Input: part model. Units: mm. Frame: model coordinates. A direction names the side the tool comes from. Give positions to 0.01 mm unless a question says otherwise; leave off trailing zeros. Write each loop counter-clockwise with the first axis right and the second up, starting at its lowest first coordinate (ties: lowest second). Pieces come first, ordered by that corner, then holes.
```python
from build123d import *

# Parameters (mm, degrees)
CROQUIS1_W                                     = 210
CROQUIS1_H                                     = 108
SALIENTE_EXTRUIR1_DEPTH                        = 103
CORTAR_EXTRUIR2_DEPTH                          = 108
REFRENTADO_PARA_TORNILLO_CON_CABEZA_2_COUNT    = 2
REFRENTADO_PARA_TORNILLO_CON_CABEZA_2_PITCH    = 76.278637259
REFRENTADO_PARA_TORNILLO_CON_CABEZA_3_COUNT    = 2
REFRENTADO_PARA_TORNILLO_CON_CABEZA_3_PITCH    = 109.392089664
REFRENTADO_PARA_TORNILLO_CON_CABEZA_4_COUNT    = 2
REFRENTADO_PARA_TORNILLO_CON_CABEZA_4_PITCH    = 78.410450701
REFRENTADO_PARA_TORNILLO_CON_CABEZA_5_AT_COUNT = 2
REFRENTADO_PARA_TORNILLO_CON_CABEZA_5_AT_PITCH = 74.028637259
REFRENTADO_PARA_TORNILLO_CON_CABEZA_6_COUNT    = 2
REFRENTADO_PARA_TORNILLO_CON_CABEZA_6_PITCH    = 111.845629414
REFRENTADO_PARA_TORNILLO_CON_CABEZA_7_COUNT    = 2
REFRENTADO_PARA_TORNILLO_CON_CABEZA_7_PITCH    = 83.840358328


# Read off the part's stored shape, not the designer's step: Refrentado para tornillo con cabeza troncocónica de #43
with BuildPart() as part:
    # Croquis1 → Saliente-Extruir1 (new body)
    with BuildSketch(Plane(origin=(0, 0, 0), x_dir=(1, 0, 0), z_dir=(0, 1, 0))):
        with Locations((105, 54)):
            Rectangle(CROQUIS1_W, CROQUIS1_H)
    extrude(amount=SALIENTE_EXTRUIR1_DEPTH)

    # Croquis2 → Cortar-Extruir2 (cut)
    with BuildSketch(Plane.XY):
        Polygon((114, 103), (210, 48.5), (210, 103), align=None)
    extrude(amount=-CORTAR_EXTRUIR2_DEPTH, mode=Mode.SUBTRACT)

    # Croquis11 → Revolución11 (revolve)
    with BuildSketch(Plane(origin=(0, 0, -54), x_dir=(-1, 0, 0), z_dir=(0, 0, -1))):
        with BuildLine():
            Line((-57, 103), (-57, 111.284271247))
            ThreePointArc((-57, 111.284271247), (-67.823922003, 109.131259298), (-77, 103))
            Line((-77, 103), (-57, 103))
        make_face()
    revolve(axis=Axis((57, 132.747407407, -54), (0, -1, 0)))

    # Croquis23 → Refrentado para tornillo con cabeza tron (revolve, cut)
    with BuildSketch(Plane(origin=(196.094171849, 56.394454523, -92.139318629), x_dir=(-0.8696333599491718, 0.49369810538781117, 0), z_dir=(0, 0, 1))):
        Polygon((0, 0), (0, 11.351936393), (2.25, 10), (2.25, 3.1), (4.5, 3.1), (4.5, 0.02875921), (4.525, 0), align=None)
    refrentado_para_tornillo_con_cabeza_tron = revolve(axis=Axis((199.229154818, 61.916626359, -92.139318629), (-0.4936981053878111, -0.8696333599491718, 0)), mode=Mode.SUBTRACT)

    # Refrentado para tornillo con cabeza  2: Refrentado para tornillo con cabeza tron ×2
    with Locations(*[(0, 0, i * REFRENTADO_PARA_TORNILLO_CON_CABEZA_2_PITCH) for i in range(1, REFRENTADO_PARA_TORNILLO_CON_CABEZA_2_COUNT)]):
        add(refrentado_para_tornillo_con_cabeza_tron, mode=Mode.SUBTRACT)

    # Refrentado para tornillo con cabeza  3: Refrentado para tornillo con cabeza tron ×2
    with Locations(*[Vector(-0.6233388895581213, 0.35387468209289175, 0.6972957321955321) * (i * REFRENTADO_PARA_TORNILLO_CON_CABEZA_3_PITCH) for i in range(1, REFRENTADO_PARA_TORNILLO_CON_CABEZA_3_COUNT)]):
        add(refrentado_para_tornillo_con_cabeza_tron, mode=Mode.SUBTRACT)

    # Refrentado para tornillo con cabeza  4: Refrentado para tornillo con cabeza tron ×2
    with Locations(*[Vector(-0.8696333599491719, 0.49369810538781106, 0) * (i * REFRENTADO_PARA_TORNILLO_CON_CABEZA_4_PITCH) for i in range(1, REFRENTADO_PARA_TORNILLO_CON_CABEZA_4_COUNT)]):
        add(refrentado_para_tornillo_con_cabeza_tron, mode=Mode.SUBTRACT)

    # Croquis26 → Refrentado para tornillo con cabeza  5 (revolve, cut)
    with BuildSketch(Plane(origin=(98.029898951, 103, -92.139318629), x_dir=(0, 0, 1), z_dir=(1, 0, 0))):
        Polygon((0, 0), (0, 11.351936393), (2.25, 10), (2.25, 3.1), (4.5, 3.1), (4.5, 0.02875921), (4.525, 0), align=None)
    refrentado_para_tornillo_con_cabeza_5 = revolve(axis=Axis((98.029898951, 109.35, -92.139318629), (0, -1, 0)), mode=Mode.SUBTRACT)

    # Refrentado para tornillo con cabeza 5 at: Refrentado para tornillo con cabeza  5 ×2
    with Locations(*[(0, 0, i * REFRENTADO_PARA_TORNILLO_CON_CABEZA_5_AT_PITCH) for i in range(1, REFRENTADO_PARA_TORNILLO_CON_CABEZA_5_AT_COUNT)]):
        add(refrentado_para_tornillo_con_cabeza_5, mode=Mode.SUBTRACT)

    # Refrentado para tornillo con cabeza  6: Refrentado para tornillo con cabeza  5 ×2
    with Locations(*[Vector(-0.7496078189874714, 0, 0.6618822536621196) * (i * REFRENTADO_PARA_TORNILLO_CON_CABEZA_6_PITCH) for i in range(1, REFRENTADO_PARA_TORNILLO_CON_CABEZA_6_COUNT)]):
        add(refrentado_para_tornillo_con_cabeza_5, mode=Mode.SUBTRACT)

    # Refrentado para tornillo con cabeza  7: Refrentado para tornillo con cabeza  5 ×2
    with Locations(*[(-i * REFRENTADO_PARA_TORNILLO_CON_CABEZA_7_PITCH, 0, 0) for i in range(1, REFRENTADO_PARA_TORNILLO_CON_CABEZA_7_COUNT)]):
        add(refrentado_para_tornillo_con_cabeza_5, mode=Mode.SUBTRACT)

    # Refrentado para tornillo con cabeza 8 ou → Refrentado para tornillo con cabeza  8 (revolve, cut)
    with BuildSketch(Plane(origin=(70, 0, -54), x_dir=(1, 0, 0), z_dir=(0, 0, 1))):
        Polygon((1.63195, 10.299425513), (0, 11.28), (0, 0), (3.175, 0), (3.175, 2.032), (1.63195, 2.032), align=None)
    revolve(axis=Axis((70, 0, -54), (0, 1, 0)), mode=Mode.SUBTRACT)

    # Refrentado para tornillo con cabeza  9 → Refrentado para tornillo con cabeza 8 2 (revolve, cut)
    with BuildSketch(Plane(origin=(50, 0, -73.797820485), x_dir=(1, 0, 0), z_dir=(0, 0, 1))):
        Polygon((0, 0), (3.175, 0), (3.175, 2.032), (1.63195, 2.032), (1.63195, 10.299425513), (0, 11.28), align=None)
    revolve(axis=Axis((50, 0, -73.797820485), (0, 1, 0)), mode=Mode.SUBTRACT)

    # Refrentado para tornillo con cabeza  10 → Refrentado para tornillo con cabeza 8 3 (revolve, cut)
    with BuildSketch(Plane(origin=(50, 0, -33.797820485), x_dir=(1, 0, 0), z_dir=(0, 0, 1))):
        Polygon((0, 0), (3.175, 0), (3.175, 2.032), (1.63195, 2.032), (1.63195, 10.299425513), (0, 11.28), align=None)
    revolve(axis=Axis((50, 0, -33.797820485), (0, 1, 0)), mode=Mode.SUBTRACT)

    # Refrentado para tornillo con cabeza  11 → Refrentado para tornillo con cabeza 8 4 (revolve, cut)
    with BuildSketch(Plane(origin=(50, 0, -53.797820485), x_dir=(1, 0, 0), z_dir=(0, 0, 1))):
        Polygon((0, 0), (3.175, 0), (3.175, 2.032), (1.63195, 2.032), (1.63195, 10.299425513), (0, 11.28), align=None)
    revolve(axis=Axis((50, 0, -53.797820485), (0, 1, 0)), mode=Mode.SUBTRACT)

    # Refrentado para tornillo con cabeza  12 → Refrentado para tornillo con cabeza 8 5 (revolve, cut)
    with BuildSketch(Plane(origin=(30, 0, -54), x_dir=(1, 0, 0), z_dir=(0, 0, 1))):
        Polygon((0, 0), (3.175, 0), (3.175, 2.032), (1.63195, 2.032), (1.63195, 10.299425513), (0, 11.28), align=None)
    revolve(axis=Axis((30, 0, -54), (0, 1, 0)), mode=Mode.SUBTRACT)


solid = part.part
```
Item 1: Pin query (flat end, axial travel): pin 1 (10 mm diameter, centred on x = 96.5, z = -16, fed in from +Y); pin 2 (3.5 mm diameter, centred on x = 14.19, z = -18.11, fed in from +Y); pin 3 (3 mm diameter, centred on x = 70.5, z = -55.5, fed in from -Y). Return the tip coordinate at first contact, or that it passes through.
Item 2: Section D-D (x = 183.5). Return loops of the section in (y, z), and give its area (3 significant figures).
Item 3: Section A-A (z = -7). Return loops of the section in (x, y).
Item 4: Set-up query: faces 1 (the flat face through (31.4, 2.032, -52.6)), 2 (the flat face through (104, 51, -108)). Return all of +Z, -Z, +X, -X, +Y, -Y with unobstructed straight access to the full face (end or side cutting, diameter ignored); none if empty.
Item 5: Ray query, line 1 (Z direction, x = 50, y = 8); line 2 (Z direction, x = 70, y = 8); line 3 (Y direction, x = 33, z = -49.5). Return the intervals inside material, ascending.
Item 6: Mould query, pull axis X, two halves, no side actions, for faces 3 (the flat face through (0, 51, -53)), 4 (the flat face through (196.25, 52.74, -90.2)), 5 (the flat face through (56, 103, -31)), 6 (the cylindrical face through (52.93, 1.03, -52.58)). Classes: +X half, -X half, draft (parallel to the pull), parting line (faces both ways), or undercut.
Item 7: Section C-C (z = -43). Return loops of the section in (x, y), and give its area (3 significant figures).
Item 8: Section B-B (x = 87). Return loops of the section in (y, z), and give its area (3 significant figures).
Solved:
1. pin 1: stops at y = 103
1. pin 2: stops at y = 92.7
1. pin 3: stops at y = 2.03
2. outline: (0, -108) - (63.54, -108) - (63.54, 0) - (0, 0) - close
2. area: 6,860 mm2
3. outline: (0, 0) - (210, 0) - (210, 48.5) - (114, 103) - (0, 103) - close
4. face 1: -Y
4. face 2: -Z, +X, -X, +Y, -Y
5. line 1: z = -108 to -75.43, -72.17 to -55.43, -52.17 to -35.43, -32.17 to 0
5. line 2: z = -108 to -55.63, -52.37 to 0
5. line 3: y = 0 to 103
6. face 3: -X half
6. face 4: undercut
6. face 5: draft
6. face 6: undercut
7. outline: (0, 0) - (210, 0) - (210, 48.5) - (114, 103) - (73.7, 103) arc R26.06 ccw to (40.3, 103) - (0, 103) - close
7. area: 19,200 mm2
8. outline: (0, -108) - (103, -108) - (103, 0) - (0, 0) - close
8. area: 11,100 mm2
